Geometry check sheet. Reference: drawing and pictorial views, mm from the part's lowest x, y, z. A direction names the side the tool comes from. Give positions to 0.01 mm unless a question says otherwise; leave off trailing zeros. Order: outer loops, then holes, each group sorted by start corner. A loop starts at its lowest first (then second) coordinate and runs counter-clockwise, first axis right, second up.
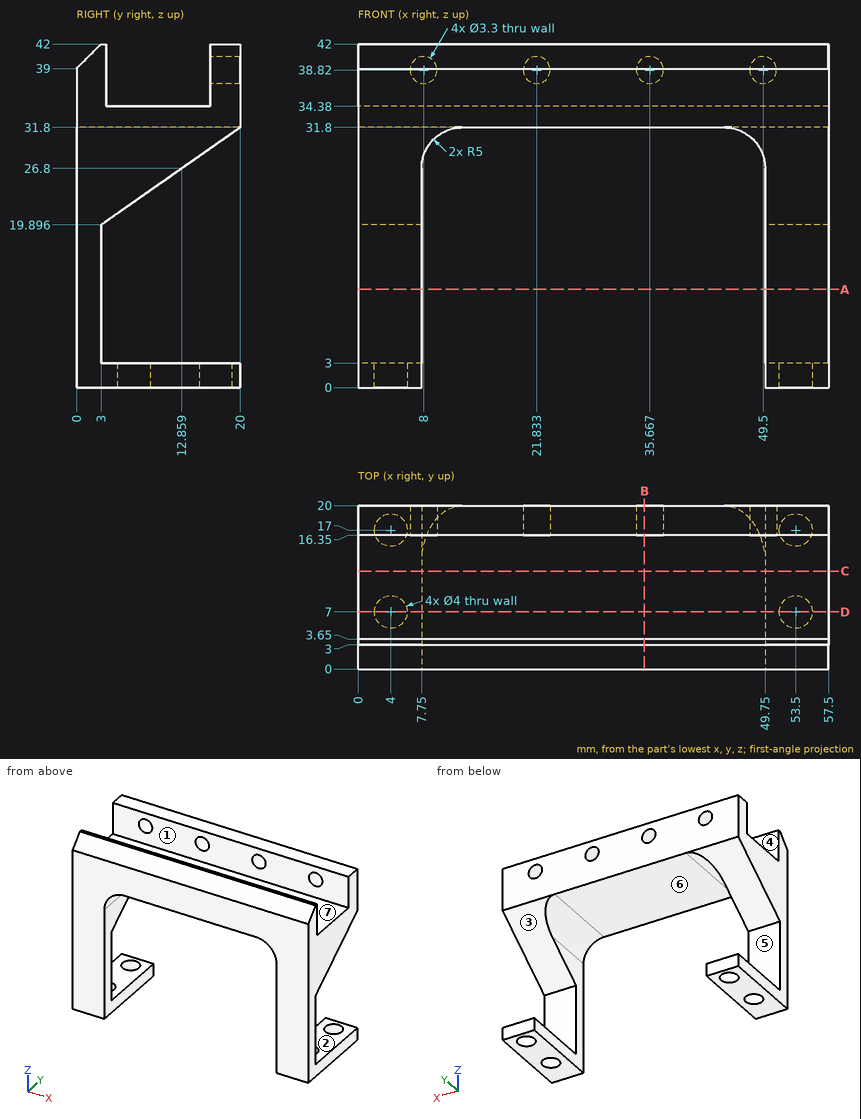
1) Depth check by flat-ended pin: pin 1 Ø2 at (x, z) = (49.5, 38.82) entering from +Y; pin 2 Ø6 at (x, y) = (3.5, 8.5) entering from +Z; pin 3 Ø3 at (x, y) = (4, 7) entering from -Z; pin 4 Ø6 at (y, z) = (8.5, 10) entering from +X. Enter the tip coordinate at first touch or a pass-through.
Recorded:
pin 1: stops at y = 3.65
pin 2: stops at z = 34.38
pin 3: stops at z = 21.65
pin 4: passes through
2) Set-up check for the marked faces 5, 6 and 7: record each of +Z, -Z, +X, -X, +Y, -Y from which the full face is reachable in a straight line by a thin tool's end or side.
Recorded:
face 5: +X, -X, +Y
face 6: -Z, +Y, -Y
face 7: +Z, +X, -X
3) Section check D-D, the plane y = 7. Record the cut outline in (x, z).
Recorded:
outline: (0, 0) - (2, 0) - (2, 3) - (0, 3) - close; (0, 22.7) - (7.75, 22.7) - (7.75, 26.8) arc R5 cw to (12.75, 31.8) - (44.75, 31.8) arc R5 cw to (49.75, 26.8) - (49.75, 22.7) - (57.5, 22.7) - (57.5, 34.38) - (0, 34.38) - close; (6, 0) - (7.75, 0) - (7.75, 3) - (6, 3) - close; (49.75, 0) - (51.5, 0) - (51.5, 3) - (49.75, 3) - close; (55.5, 0) - (57.5, 0) - (57.5, 3) - (55.5, 3) - close
4) Draft check along Y on the marked faces 1, 2, 3 and 4. Enter one of: +Y half, -Y half, draft (parallel to the pull), parting line (faces both ways), or undercut.
Recorded:
face 1: undercut
face 2: draft
face 3: +Y half
face 4: undercut
5) Material ranges on L1, parallel to Y at x = 53.5, z = 1.4; L2, parallel to X at y = 18.45, z = 38.82; L3, parallel to Y at x = 53, z = 2, recorded low to high.
Recorded:
L1: y = 0 to 5, 9 to 15, 19 to 20
L2: x = 0 to 6.35, 9.65 to 20.18, 23.48 to 34.02, 37.32 to 47.85, 51.15 to 57.5
L3: y = 0 to 5.06, 8.94 to 15.06, 18.94 to 20
6) Section check A-A, the plane z = 12. Record the cut outline in (x, y).
Recorded:
outline: (0, 0) - (7.75, 0) - (7.75, 3) - (0, 3) - close; (49.75, 0) - (57.5, 0) - (57.5, 3) - (49.75, 3) - close
7) Section check B-B, the plane x = 35. Record the cut outline in (y, z).
Recorded:
outline: (0, 31.8) - (20, 31.8) - (20, 37.31) - (16.35, 37.31) - (16.35, 34.38) - (3.65, 34.38) - (3.65, 42) - (3, 42) - (0, 39) - close; (16.35, 40.33) - (20, 40.33) - (20, 42) - (16.35, 42) - close
8) Section check C-C, the plane y = 12. Record the cut outline in (x, z).
Recorded:
outline: (0, 0) - (7.75, 0) - (7.75, 3) - (0, 3) - close; (0, 26.2) - (7.75, 26.2) - (7.75, 26.8) arc R5 cw to (12.75, 31.8) - (44.75, 31.8) arc R5 cw to (49.75, 26.8) - (49.75, 26.2) - (57.5, 26.2) - (57.5, 34.38) - (0, 34.38) - close; (49.75, 0) - (57.5, 0) - (57.5, 3) - (49.75, 3) - close
